from build123d import *

# Parameters (mm, degrees)
F1_DEPTH = 1.5
F3_DEPTH = 1.501
F4_R     = 4.5
F5_DEPTH = 3
F6_R     = 2.5
F7_DEPTH = 2.5
F8_R     = 2.49999


# Not quite as in the source:
# - a fillet or chamfer is up to 0.001 mm smaller than in the source, because OpenCascade refuses the exact size


with BuildPart() as f1:
    # F0 (on Top) → F1 (new body)
    with BuildSketch(Plane.XY):
        Polygon((9.95, -5.7446351784), (9.95, 5.7446351784), (0, 11.4892703569), (-9.95, 5.7446351784), (-9.95, -5.7446351784), (0, -11.4892703569), align=None)
    extrude(amount=F1_DEPTH)

    # F2 (on face) → F3 (cut, through all)
    with BuildSketch(Plane.XY.offset(1.5)):
        with BuildLine():
            Line((-1.6, 10.5655099262), (-1.6, 9.5))
            ThreePointArc((-1.6, 9.5), (0, 7.9), (1.6, 9.5))
            Line((1.6, 9.5), (1.6, 10.5655099262))
            Line((1.6, 10.5655099262), (0, 11.4892703569))
            Line((0, 11.4892703569), (-1.6, 10.5655099262))
        make_face()
        with BuildLine():
            Line((9.95, 5.7446351784), (8.35, 6.6683956091))
            Line((8.35, 6.6683956091), (7.427241336, 6.1356406461))
            ThreePointArc((7.427241336, 6.1356406461), (6.8416006899, 3.95), (9.027241336, 3.3643593539))
            Line((9.027241336, 3.3643593539), (9.95, 3.897114317))
            Line((9.95, 3.897114317), (9.95, 5.7446351784))
        make_face()
        with BuildLine():
            Line((9.95, -5.7446351784), (9.95, -3.897114317))
            Line((9.95, -3.897114317), (9.027241336, -3.3643593539))
            ThreePointArc((9.027241336, -3.3643593539), (6.8416006899, -3.95), (7.427241336, -6.1356406461))
            Line((7.427241336, -6.1356406461), (8.35, -6.6683956091))
            Line((8.35, -6.6683956091), (9.95, -5.7446351784))
        make_face()
        with BuildLine():
            Line((-9.027241336, -3.3643593539), (-9.95, -3.897114317))
            Line((-9.95, -3.897114317), (-9.95, -5.7446351784))
            Line((-9.95, -5.7446351784), (-8.35, -6.6683956091))
            Line((-8.35, -6.6683956091), (-7.427241336, -6.1356406461))
            ThreePointArc((-7.427241336, -6.1356406461), (-6.8416006899, -3.95), (-9.027241336, -3.3643593539))
        make_face()
        with BuildLine():
            Line((-7.427241336, 6.1356406461), (-8.35, 6.6683956091))
            Line((-8.35, 6.6683956091), (-9.95, 5.7446351784))
            Line((-9.95, 5.7446351784), (-9.95, 3.897114317))
            Line((-9.95, 3.897114317), (-9.027241336, 3.3643593539))
            ThreePointArc((-9.027241336, 3.3643593539), (-6.8416006899, 3.95), (-7.427241336, 6.1356406461))
        make_face()
        with BuildLine():
            Line((-1.6, -9.5), (-1.6, -10.5655099262))
            Line((-1.6, -10.5655099262), (0, -11.4892703569))
            Line((0, -11.4892703569), (1.6, -10.5655099262))
            Line((1.6, -10.5655099262), (1.6, -9.5))
            ThreePointArc((1.6, -9.5), (0, -7.9), (-1.6, -9.5))
        make_face()
    extrude(amount=-F3_DEPTH, mode=Mode.SUBTRACT)

    # F4 (on face) → F5 (join)
    with BuildSketch(Plane.XY.offset(1.5)):
        Circle(F4_R)
    extrude(amount=F5_DEPTH)

    # F6 (on face) → F7 (join)
    with BuildSketch(Plane.XY.offset(4.5)):
        Circle(F6_R)
    extrude(amount=F7_DEPTH)

    # F8 (radius 2.5 in the source; OpenCascade refuses exactly that, so slightly less here)
    f8_edges = [f1.edges().sort_by_distance(p)[0] for p in [
        (-2.5, 0, 7),
    ]]
    fillet(f8_edges, radius=F8_R)


solid = f1.part
Model file for the job. Use its own axes, mm. A direction names the side the tool comes from. Round coordinates to 2 decimals unless told otherwise and drop trailing zeros. Order: outer loops, then holes, each group sorted by start corner. A loop starts at its lowest first (then second) coordinate and runs counter-clockwise, first axis right, second up.
(1) Band-saw the part on B-B (z = 4). List the corners of the cut face in (x, y).
(2) Band-saw the part on A-A (y = 4.75). List the corners of the cut face in (x, z).
(3) Pull direction Y, two halves, no side cores. Call faces 1 (the face through (0, -7.9, 0.8)), 2 (the face through (9.95, 0, 1)), 3 (the face through (7.882, -6.398, 0.76)), 4 (the face through (5.02, 8.59, 0.74)): released by +Y, released by -Y, zero draft, split by the parting line, or undercut.
(4) 3-axis set-ups, long thin cutter, end or side, ignore diameter. For faces 5 (the face through (-9.95, 0, 1)), 6 (the face through (-5, 0, 1.5)), 7 (the face through (9.495, -3.634, 0.76)), 8 (the face through (-9.495, 3.634, 0.76)), 9 (the face through (-7.9, -6.41, 0.76)): which of +Z, -Z, +X, -X, +Y, -Y reach the whole face in a straight line?
(5) Pin check, flat tips, straight feed: pin 1 (0.9 mm diameter, centred on y = -10, z = 0.5, fed in from +X); pin 2 (1 mm diameter, centred on x = 4.5, z = 3, fed in from +Y); pin 3 (1.5 mm diameter, centred on x = -1.5, z = 4, fed in from -Y). Stop position of each tip, or through.
(6) Drill centre lines: line 1 (Z direction, x = -4.25, y = -4.75); line 2 (Z direction, x = -1.25, y = 3); line 3 (X direction, y = -9.25, z = 0.75). Where is each one in solid material? Low to high.
(7) Band-saw the part on C-C (x = 5.5). List the corners of the cut face in (y, z), then the cut area to 3 significant figures.
Verdict:
1. outline: circle Ø9 at (0, 0)
2. outline: (-6.63, 0) - (6.63, 0) - (6.63, 1.5) - (-6.63, 1.5) - close
3. face 1: released by -Y
3. face 2: zero draft
3. face 3: undercut
3. face 4: released by +Y
4. face 5: +Z, -Z, -X, +Y, -Y
4. face 6: +Z
4. face 7: +Z, -Z, -Y
4. face 8: +Z, -Z, +Y
4. face 9: +Z, -Z, -X
5. pin 1: stops at x = 3.36
5. pin 2: stops at y = 2.06
5. pin 3: stops at y = -4.44
6. line 1: z = 0 to 1.5
6. line 2: z = 0 to 4.5
6. line 3: x = -3.88 to -1.58, 1.58 to 3.88
7. outline: (-8.31, 0) - (8.31, 0) - (8.31, 1.5) - (-8.31, 1.5) - close
7. area: 24.9 mm2
